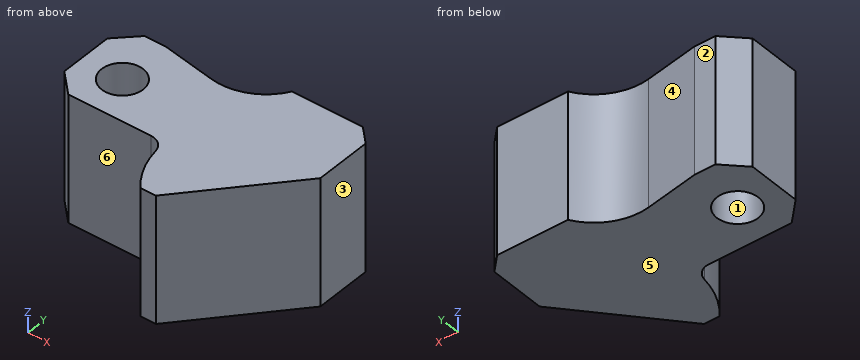
```python
from build123d import *

# Parameters (mm, degrees)
ESQUISSE2_R        = 7
BOSS_EXTRU_2_DEPTH = 21.5


with BuildPart() as part:
    # Esquisse2 → Boss.-Extru.2 (new body, symmetric)
    with BuildSketch(Plane.XY):
        with BuildLine():
            Line((46.788067397, -19), (52, -19))
            Line((52, -19), (81, 14))
            Line((81, 14), (81, 33))
            Line((81, 33), (76, 38))
            Line((76, 38), (52, 38))
            ThreePointArc((52, 38), (43.513473837, 30.283893076), (32.139737934, 28.801474779))
            Line((32.139737934, 28.801474779), (14, 32))
            Line((14, 32), (7, 32))
            Line((7, 32), (0, 25))
            Line((0, 25), (0, 7))
            Line((0, 7), (7, 0))
            Line((7, 0), (35.066626255, 0))
            ThreePointArc((35.066626255, 0), (38.331862036, -1.213413768), (40.012264997, -4.264705882))
            ThreePointArc((40.012264997, -4.264705882), (42.3490952, -12.115672061), (46.788067397, -19))
        make_face()
        with Locations((14, 14)):
            Circle(ESQUISSE2_R, mode=Mode.SUBTRACT)
    extrude(amount=BOSS_EXTRU_2_DEPTH, both=True)


solid = part.part
```
Geometry: final body of the model. Coordinates: model frame, mm. Face numbers are marked on the shaded views. A direction names the side the tool comes from. Coordinates: 2 decimals unless noted, no trailing zeros. Loops run counter-clockwise (first coordinate to the right, second up) from the corner with the lowest first, then second, coordinate; pieces in that order, holes last. Notation, with made-up numbers: (59.5, 87) -> (78.5, 87) arc R10 ccw to (78.5, 100) -> close; hole circle Ø4 at (69, -13). An arc over 180 degrees is marked (long way). Use a Markdown table: item, result. Add a question column.
(1) Section query A-A, the plane z = -15. Return loops of the section in (x, y).
(2) Mould query, pull axis X, two halves, no side actions, for the marked faces 1, 2 and 3. Classes: pulls with the +X half, pulls with the -X half, needs draft (parallel to the pull), parting line crosses it, or undercut.
(3) Section query D-D, the plane y = 34.5. Return loops of the section in (x, z), plus the area to 3 significant figures.
(4) Access query for the marked faces 4, 5 and 6. Directions: +Z, -Z, +X, -X, +Y, -Y. A direction counts if a zero-diameter tool reaches every point of the face in a straight line with its end or side. Return the directions, or none.
(5) Pin query (flat end, axial travel): pin 1 Ø22.5 at (x, z) = (20, -5) entering from -Y; pin 2 Ø7.5 at (x, z) = (9, -10.5) entering from +Y; pin 3 Ø12 at (x, z) = (70.5, 16.5) entering from -Y. Return the tip coordinate at first contact, or that it passes through.
(6) Section query C-C, the plane y = 9. Return loops of the section in (x, z).
(7) Line query: line 1 along Y through (x, z) = (14, -2); line 2 along X through (y, z) = (16, 16); line 3 along X through (y, z) = (9, -8). Output: solid intervals per line, ascending.
(8) Section query B-B, the plane x = 19. Return loops of the section in (y, z), plus the area to 3 significant figures.
Answer:
| question | item | result |
|---|---|---|
| 1 | outline | (0, 7) -> (7, 0) -> (35.07, 0) arc R5 cw to (40.01, -4.26) arc R29 ccw to (46.79, -19) -> (52, -19) -> (81, 14) -> (81, 33) -> (76, 38) -> (52, 38) arc R19.15 cw to (32.14, 28.8) -> (14, 32) -> (7, 32) -> (0, 25) -> close; hole circle Ø14 at (14, 14) |
| 2 | face 1 | undercut |
| 2 | face 2 | needs draft |
| 2 | face 3 | pulls with the +X half |
| 3 | outline | (49.38, -21.5) -> (79.5, -21.5) -> (79.5, 21.5) -> (49.38, 21.5) -> close |
| 3 | area | 1,300 mm^2 |
| 4 | face 4 | +Z, -Z, +Y |
| 4 | face 5 | -Z, +X, -X, +Y, -Y |
| 4 | face 6 | +Z, -Z, -X, -Y |
| 5 | pin 1 | stops at y = 0 |
| 5 | pin 2 | stops at y = 32 |
| 5 | pin 3 | stops at y = -4.78 |
| 6 | outline | (0, -21.5) -> (9.1, -21.5) -> (9.1, 21.5) -> (0, 21.5) -> close; (18.9, -21.5) -> (76.61, -21.5) -> (76.61, 21.5) -> (18.9, 21.5) -> close |
| 7 | line 1 | y = 0 to 7, 21 to 32 |
| 7 | line 2 | x = 0 to 7.29, 20.71 to 81 |
| 7 | line 3 | x = 0 to 9.1, 18.9 to 76.61 |
| 8 | outline | (0, -21.5) -> (9.1, -21.5) -> (9.1, 21.5) -> (0, 21.5) -> close; (18.9, -21.5) -> (31.12, -21.5) -> (31.12, 21.5) -> (18.9, 21.5) -> close |
| 8 | area | 917 mm^2 |
